Could you check a few things on this model? Use its own coordinates, in mm. A direction names the side the tool comes from. Give positions to 0.01 mm unless a question says otherwise; leave off trailing zeros. Write each loop counter-clockwise with the first axis right and the second up, starting at its lowest first coordinate (ties: lowest second). Pieces come first, ordered by that corner, then holes. Notation, with made-up numbers: (28.5, 48.5) -> (35.5, 48.5) arc R17 cw to (35.5, 60.5) -> close; hole circle Ø5 at (68, 18.5). An arc over 180 degrees is marked (long way). One line per question, with ' | ' between items.
from build123d import *

# Parameters (mm, degrees)
SKETCH_1_W           = 37
SKETCH_1_H           = 628.32
EXTRUDE_1_DEPTH      = 3
SKETCH_2_W           = 5
SKETCH_2_H           = 628.32
EXTRUDE_2_DEPTH      = 10
EXTRUDE_2_DEPTH_BACK = 3
SKETCH_3_R           = 2.6
CUT_EXTRUDE_1_DEPTH  = 10
EXTRUDE_3_DEPTH      = 628.32


with BuildPart() as part:
    # 스케치1 → 보스-돌출1 (new body)
    with BuildSketch(Plane(origin=(0, 0, 0), x_dir=(1, 0, 0), z_dir=(0, 1, 0))):
        with Locations((-18.5, -314.16)):
            Rectangle(SKETCH_1_W, SKETCH_1_H)
    extrude(amount=EXTRUDE_1_DEPTH)

    # 스케치2 → 보스-돌출2 (add, two sides)
    with BuildSketch(Plane.XZ) as extrude_2_sk:
        with Locations((2.5, 314.16)):
            Rectangle(SKETCH_2_W, SKETCH_2_H)
    extrude(amount=EXTRUDE_2_DEPTH)
    extrude(extrude_2_sk.sketch, amount=-EXTRUDE_2_DEPTH_BACK)

    # 스케치3 → 컷-돌출1 (cut)
    with BuildSketch(Plane.XZ):
        with Locations((-27, 40)):
            Circle(SKETCH_3_R)
        with Locations((-27, 80)):
            Circle(SKETCH_3_R)
        with Locations((-27, 120)):
            Circle(SKETCH_3_R)
        with Locations((-27, 160)):
            Circle(SKETCH_3_R)
        with Locations((-27, 200)):
            Circle(SKETCH_3_R)
        with Locations((-27, 240)):
            Circle(SKETCH_3_R)
        with Locations((-27, 280)):
            Circle(SKETCH_3_R)
        with Locations((-27, 320)):
            Circle(SKETCH_3_R)
        with Locations((-27, 360)):
            Circle(SKETCH_3_R)
        with Locations((-27, 400)):
            Circle(SKETCH_3_R)
        with Locations((-27, 440)):
            Circle(SKETCH_3_R)
        with Locations((-27, 480)):
            Circle(SKETCH_3_R)
        with Locations((-27, 520)):
            Circle(SKETCH_3_R)
        with Locations((-27, 560)):
            Circle(SKETCH_3_R)
        with Locations((-27, 600)):
            Circle(SKETCH_3_R)
        with Locations((-27, 640)):
            Circle(SKETCH_3_R)
    extrude(amount=-CUT_EXTRUDE_1_DEPTH, mode=Mode.SUBTRACT)

    # 스케치4 → 보스-돌출3 (add)
    with BuildSketch(Plane.XY.offset(628.32)):
        Polygon((0, 0), (0, -6), (-6, 0), align=None)
    extrude(amount=-EXTRUDE_3_DEPTH)


solid = part.part
Q1. On a 3-axis mill with a long thin cutter (end or side, diameter ignored), from which of +Z, -Z, +X, -X, +Y, -Y can I reach the whole of each face in a straight line? I mean faces 1 (the flat face through (-22, 0, 310)), 2 (the flat face through (-10, 1, 0)). Say none if no direction works.
Answer below:
face 1: +Z, -Z, -X, -Y | face 2: -Z, +X, -X, +Y, -Y
Q2. Will these pins go through, and if not, where does the flat tip stop? pin 1 (7 mm diameter, centred on x = -27, z = 520, fed in from -Y); pin 2 (3 mm diameter, centred on y = -8, z = 259.5, fed in from -X).
Answer below:
pin 1: stops at y = 0 | pin 2: stops at x = 0
Q3. Imagine slicing it at A-A on z = 431. Please give me the cut outline in (x, y).
Answer below:
outline: (-37, 0) -> (-6, 0) -> (0, -6) -> (0, -10) -> (5, -10) -> (5, 3) -> (-37, 3) -> close
Q4. If I drill on line 1 along X through (y, z) = (1.2, 480); line 2 along Y through (x, z) = (-22.5, 48); line 3 along X through (y, z) = (-6, 167.5), over which ranges is the centre line in solid material (lowest first)?
Answer below:
line 1: x = -37 to -29.6, -24.4 to 5 | line 2: y = 0 to 3 | line 3: x = 0 to 5
Q5. Imagine slicing it at B-B on x = -18. Please give me the cut outline in (y, z), and give its area (3 significant figures).
Answer below:
outline: (0, 0) -> (3, 0) -> (3, 628.32) -> (0, 628.32) -> close | area: 1,880 mm^2
